Can you work these out from the model? Positions are in its coordinate system, mm. A direction names the side the tool comes from. Give positions to 0.01 mm unless a question says otherwise; leave off trailing zeros. Order: outer loops, then holes, each group sorted by start corner. A loop starts at its lowest first (then second) coordinate and runs counter-clockwise, first axis right, second up.
Item 1: If we mould it in two halves opening along Z, with no side actions, what happens to faces 1 (the flat face through (0, 48, -1.6)), 2 (the flat face through (-21, 19, 0)), 3 (the cylindrical face through (-15.869, 34.958, 16.673))? For each: +Z half, -Z half, draft (parallel to the pull), parting line (faces both ways), or undercut.
Item 2: I want a section at C-C, the plane y = 36. Write out the boundary of the cut face in (x, z).
Item 3: I want a section at A-A, the plane z = 15.5. Write out the boundary of the cut face in (x, y).
Item 4: I want a section at B-B, the plane x = 0. Write out the boundary of the cut face in (y, z).
Item 5: Which directions (+Z, -Z, +X, -X, +Y, -Y) give clear straight access to the entire face, cutting with the end or side of a thin tool? Please do faces 4 (the flat face through (0, 48, 1.6)), 5 (the cylindrical face through (-19.717, 18.734, -19.647)), 6 (the flat face through (1.6, 48, 0)), 7 (the flat face through (-16, 32, -16)).
Item 6: I want a section at D-D, the plane z = 0. Write out the boundary of the cut face in (x, y), then the cut area to 3 significant figures.
Item 7: If I drill on line 1 along X through (y, z) = (36.4, -15.5); line 2 along X through (y, z) = (35, 15), over which ranges is the centre line in solid material (lowest first)?
Item 8: I'm going to push flat-ended pins straight in: pin 1 Ø0.7 at (x, z) = (-15.5, 15.5) entering from +Y; pin 2 Ø1.2 at (x, z) = (15, -15) entering from +Y; pin 3 Ø3.5 at (y, z) = (50, 0.5) entering from +X. Where does each tip first touch, or does it pass through?
Autodesk Inventor part; units mm, degrees
ref_plane "YZ Plane" through (0, 0, 0) normal (1, 0, 0) x (0, 1, 0)
ref_plane "XZ Plane" through (0, 0, 0) normal (0, 1, 0) x (-1, 0, 0)
ref_plane "XY Plane" through (0, 0, 0) normal (0, 0, 1) x (1, 0, 0)
sketch "Sketch1" plane through (0, 0, 0) normal (0, 1, 0) x (-1, 0, 0)
  line L0 (-16.5, -21) -> (16.5, -21)
  line L1 (21, -16.5) -> (21, 16.5)
  line L2 (16.5, 21) -> (-16.5, 21)
  line L3 (-21, 16.5) -> (-21, -16.5)
  line L4 (-21, -21) -> (21, 21) construction
  line L5 (21, -21) -> (-21, 21) construction
  arc A0 (21, 16.5) -> (16.5, 21) centre (16.5, 16.5) ccw
  arc A1 (-16.5, 21) -> (-21, 16.5) centre (-16.5, 16.5) ccw
  arc A2 (-21, -16.5) -> (-16.5, -21) centre (-16.5, -16.5) ccw
  arc A3 (16.5, -21) -> (21, -16.5) centre (16.5, -16.5) ccw
  point P0 (0, 0)
  dimension "d0" = 42
  dimension "d1" = 42
  dimension "d2" = 4.5
extrude "Extrusion1" add sketch "Sketch1" along normal blind 38
sketch "Sketch2" plane through (0, 38, 0) normal (0, 1, 0) x (1, 0, 0)
  circle A0 centre (0, 0) radius 11
  dimension "d5" = 22
extrude "Extrusion2" add sketch "Sketch2" along normal blind 2
sketch "Sketch3" plane through (0, 38, 0) normal (0, 1, 0) x (1, 0, 0)
  line L0 (-15.5, -15.5) -> (15.5, -15.5) construction
  line L1 (15.5, -15.5) -> (15.5, 15.5) construction
  line L2 (15.5, 15.5) -> (-15.5, 15.5) construction
  line L3 (-15.5, 15.5) -> (-15.5, -15.5) construction
  line L4 (-15.5, -15.5) -> (15.5, 15.5) construction
  line L5 (15.5, -15.5) -> (-15.5, 15.5) construction
  point P0 (0, 0)
  dimension "d8" = 31
  dimension "d9" = 31
hole "Hole1" at (-15.5, 38, 15.5) at (-15.5, 38, -15.5) at (15.5, 38, -15.5) at (15.5, 38, 15.5) direction (0, -1, 0) diameter 2.459 depth 6
sketch "Sketch4" plane through (0, 40, 0) normal (0, 1, 0) x (1, 0, 0)
  circle A0 centre (0, 0) radius 2.5
  dimension "d17" = 5
extrude "Extrusion3" add sketch "Sketch4" along normal blind 3.4
sketch "Sketch5" plane through (0, 43.4, 0) normal (0, 1, 0) x (1, 0, 0)
  line L0 (1.6, -1.6) -> (-1.6, -1.6)
  line L1 (-1.6, -1.6) -> (-1.6, 1.6)
  line L2 (-1.6, 1.6) -> (1.6, 1.6)
  line L3 (1.6, 1.6) -> (1.6, -1.6)
  circle A0 centre (0, 0) radius 2.5 construction
  line L4 (1.6, -1.6) -> (-1.6, 1.6) construction
  line L5 (-1.6, -1.6) -> (1.6, 1.6) construction
  circle A1 centre (0, 0) radius 2.5 construction
  circle A2 centre (0, 0) radius 11
  dimension "d20" = 3.2
  dimension "d21" = 3.2
extrude "Extrusion4" add sketch "Sketch5" along normal blind 8.6 contours L0 L1 L2 L3
properties part number "stepper"
Results list:
1. face 1: -Z half
1. face 2: draft
1. face 3: undercut
2. outline: (-21, -16.5) arc R4.5 ccw to (-16.5, -21) - (16.5, -21) arc R4.5 ccw to (21, -16.5) - (21, 16.5) arc R4.5 ccw to (16.5, 21) - (-16.5, 21) arc R4.5 ccw to (-21, 16.5) - close; hole circle Ø2.46 at (-15.5, -15.5); hole circle Ø2.46 at (-15.5, 15.5); hole circle Ø2.46 at (15.5, -15.5); hole circle Ø2.46 at (15.5, 15.5)
3. outline: (-21, 0) - (21, 0) - (21, 38) - (16.73, 38) - (16.73, 32) - (14.27, 32) - (14.27, 38) - (-14.27, 38) - (-14.27, 32) - (-16.73, 32) - (-16.73, 38) - (-21, 38) - close
4. outline: (0, -21) - (38, -21) - (38, -11) - (40, -11) - (40, -2.5) - (43.4, -2.5) - (43.4, -1.6) - (52, -1.6) - (52, 1.6) - (43.4, 1.6) - (43.4, 2.5) - (40, 2.5) - (40, 11) - (38, 11) - (38, 21) - (0, 21) - close
5. face 4: +Z, +X, -X, +Y
5. face 5: -Z, -X, +Y, -Y
5. face 6: +Z, -Z, +X, +Y
5. face 7: +Y
6. outline: (-21, 0) - (21, 0) - (21, 38) - (11, 38) - (11, 40) - (2.5, 40) - (2.5, 43.4) - (1.6, 43.4) - (1.6, 52) - (-1.6, 52) - (-1.6, 43.4) - (-2.5, 43.4) - (-2.5, 40) - (-11, 40) - (-11, 38) - (-21, 38) - close
6. area: 1,680 mm2
7. line 1: x = -21 to -16.73, -14.27 to 14.27, 16.73 to 21
7. line 2: x = -21 to -16.62, -14.38 to 14.38, 16.62 to 21
8. pin 1: stops at y = 32
8. pin 2: stops at y = 38
8. pin 3: stops at x = 1.6
